from build123d import *

# Parameters (mm, degrees)
SKETCH_F_W                   = 449
SKETCH_F_H                   = 79
SKETCH_F_R                   = 3.25
ESTRUSIONE_ESTRUSIONE1_DEPTH = 5
F_4_0_4_DIAMETER_HOLE1_D     = 4
SKETCH5_R                    = 27.5
CUT_EXTRUDE1_DEPTH           = 6


with BuildPart() as part:
    # f → Estrusione-Estrusione1 (new body)
    with BuildSketch(Plane.XY):
        with Locations((224.5, 39.5)):
            Rectangle(SKETCH_F_W, SKETCH_F_H)
        with Locations((11.5, 67.5)):
            Circle(SKETCH_F_R, mode=Mode.SUBTRACT)
        with Locations((437.5, 67.5)):
            Circle(SKETCH_F_R, mode=Mode.SUBTRACT)
        with Locations((11.5, 11.5)):
            Circle(SKETCH_F_R, mode=Mode.SUBTRACT)
        with Locations((437.5, 11.5)):
            Circle(SKETCH_F_R, mode=Mode.SUBTRACT)
    extrude(amount=ESTRUSIONE_ESTRUSIONE1_DEPTH)

    # Ø4.0 (4) Diameter Hole1 (through all)
    with Locations(Plane(origin=(0, 0, 0), x_dir=(-1, 0, 0), z_dir=(0, 0, -1))):
        with Locations((-249.5, 64.5), (-199.5, 64.5), (-249.5, 14.5), (-199.5, 14.5)):
            Hole(F_4_0_4_DIAMETER_HOLE1_D / 2)

    # Sketch5 → Cut-Extrude1 (cut, through all)
    with BuildSketch(Plane(origin=(0, 0, 0), x_dir=(-1, 0, 0), z_dir=(0, 0, -1))):
        with Locations((-224.5, 39.5)):
            Circle(SKETCH5_R)
    extrude(amount=-CUT_EXTRUDE1_DEPTH, mode=Mode.SUBTRACT)


solid = part.part
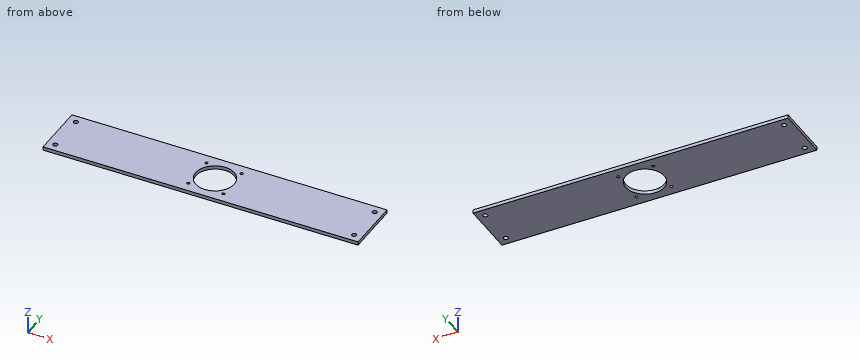
The listing builds one solid part. Answer for the finished solid, in the listing's coordinates (mm). Give positions to 0.01 mm unless a question says otherwise; leave off trailing zeros. Order: outer loops, then holes, each group sorted by start corner. A loop starts at its lowest first (then second) coordinate and runs counter-clockwise, first axis right, second up. Notation, with made-up numbers: (0.5, -5) - (41.5, -5) arc R9 cw to (41.5, 9) - close; hole circle Ø3 at (61.5, 49). An arc over 180 degrees is marked (long way). Answer as CSV lines item,"result".
Q1. Straight lines are drawn through the part: L1, parallel to Y at x = 11.5, z = 2; L2, parallel to X at y = 69, z = 3.9; L3, parallel to X at y = 21.5, z = 0.7. For each, find the intervals that lie inside material, in ascending order.
Answer key:
L1,"y = 0 to 8.25, 14.75 to 64.25, 70.75 to 79"
L2,"x = 0 to 8.62, 14.38 to 434.62, 440.38 to 449"
L3,"x = 0 to 203.71, 245.29 to 449"
Q2. A cutting plane is placed at C-C, the plane z = 4.2. Count the separate pieces of the cut face and the enclosed holes in it, and give its area (3 significant figures).
Answer key:
separate pieces,"1"
enclosed holes,"9"
area,"32,900 mm^2"
Q3. A cutting plane is placed at A-A, the plane x = 224.5. Determine the outline of the cut face in (y, z), and give its area (3 significant figures).
Answer key:
outline,"(0, 0) - (12, 0) - (12, 5) - (0, 5) - close; (67, 0) - (79, 0) - (79, 5) - (67, 5) - close"
area,"120 mm^2"
Q4. A cutting plane is placed at B-B, the plane y = 39.5. Determine the outline of the cut face in (x, z).
Answer key:
outline,"(0, 0) - (197, 0) - (197, 5) - (0, 5) - close; (252, 0) - (449, 0) - (449, 5) - (252, 5) - close"
Q5. This flat-tipped pin is pushed along its axis until it touches: pin 1 Ø5 at (x, y) = (437.5, 11.5) entering from -Z. Where does it stop, or does it pass through?
Answer key:
pin 1,"passes through"
